Work out the finished part from the listing and answer in its coordinate system (mm). Face numbers are marked on the shaded views. A direction names the side the tool comes from. Coordinates: 2 decimals unless noted, no trailing zeros. Write each loop counter-clockwise with the first axis right and the second up, starting at its lowest first coordinate (ties: lowest second). Pieces come first, ordered by that corner, then holes. Notation, with made-up numbers: M -4.5,-39.75 L 29.5,-39.75 A31 ccw 29.5,-15.75 Z; hole C 4,21 d10. An arc over 180 degrees is marked long. Use CSV: the item, a comma, the result in double quotes.
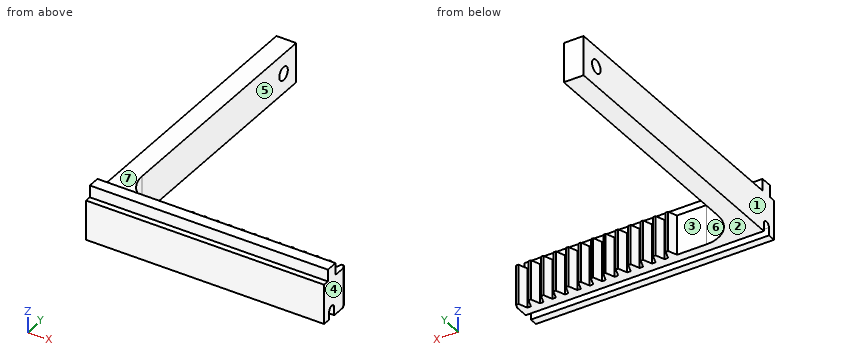
from build123d import *

# Parameters (mm, degrees)
BLANKSKE_W          = 40
BLANKSKE_H          = 8.5
BLANK_DEPTH         = 10
TOOTHCUTSIM_DEPTH   = 43.09809972
TEETHCUTS_COUNT     = 14
TEETHCUTS_PITCH     = 3.14159265
BOSS_EXTRUDE1_DEPTH = 10
SKETCH2_W           = 3
SKETCH2_H           = 3
BOSS_EXTRUDE2_DEPTH = 60
CUT_EXTRUDE2_DEPTH  = 97.566039579
MOVE_FACE2_BY       = 5
FILLET2_R           = 8
SKETCH3_R           = 1.675
CUT_EXTRUDE1_DEPTH  = 94.541434669


with BuildPart() as part:
    # BlankSke → Blank (new body)
    with BuildSketch(Plane.XY):
        with Locations((20, 4.25)):
            Rectangle(BLANKSKE_W, BLANKSKE_H)
    extrude(amount=-BLANK_DEPTH)

    # TooCutSkeSim → ToothCutSim (cut, through all)
    with BuildSketch(Plane.XY):
        Polygon((0.44443537, 6.25), (-0.44443537, 6.25), (-1.272613241, 8.5254), (1.272613241, 8.5254), align=None)
    toothcutsim = extrude(amount=-TOOTHCUTSIM_DEPTH, mode=Mode.SUBTRACT)

    # TeethCuts: ToothCutSim ×14
    with Locations(*[(i * TEETHCUTS_PITCH, 0, 0) for i in range(1, TEETHCUTS_COUNT)]):
        add(toothcutsim, mode=Mode.SUBTRACT)

    # Sketch1 → Boss-Extrude1 (add)
    with BuildSketch(Plane.XY):
        Polygon((0, 0), (-20, 0), (-20, 75), (-10, 75), (-10, 6.25), (0, 6.25), align=None)
    extrude(amount=-BOSS_EXTRUDE1_DEPTH)

    # Sketch2 → Boss-Extrude2 (add)
    with BuildSketch(Plane(origin=(40, 0, 0), x_dir=(0, 0, -1), z_dir=(1, 0, 0))):
        with Locations((-1.5, 3)):
            Rectangle(SKETCH2_W, SKETCH2_H)
    extrude(amount=-BOSS_EXTRUDE2_DEPTH)

    # Sketch5 → Cut-Extrude2 (cut, through all)
    with BuildSketch(Plane(origin=(40, 0, 0), x_dir=(0, 0, -1), z_dir=(1, 0, 0))):
        with BuildLine():
            Line((10, 4), (8, 4))
            ThreePointArc((8, 4), (7, 3), (8, 2))
            Line((8, 2), (10, 2))
            Line((10, 2), (10, 4))
        make_face()
    extrude(amount=-CUT_EXTRUDE2_DEPTH, mode=Mode.SUBTRACT)

    # Move Face2: a face moved inward by 5.0
    extrude(part.faces().sort_by_distance((-10, 40.625, -5))[0], amount=MOVE_FACE2_BY, dir=(-1, 0, 0), mode=Mode.SUBTRACT)

    # Fillet2
    fillet2_edges = [part.edges().sort_by_distance(p)[0] for p in [
        (-15, 6.25, -5),
    ]]
    fillet(fillet2_edges, radius=FILLET2_R)

    # Sketch3 → Cut-Extrude1 (cut, through all)
    with BuildSketch(Plane.ZY.offset(15)):
        with Locations(Location((-5, 70, 0), (0, 0, 90))):
            Circle(SKETCH3_R)
    extrude(amount=CUT_EXTRUDE1_DEPTH, mode=Mode.SUBTRACT)


solid = part.part
Item 1: Consider probe 1 along Z at (x, y) = (-16.65, 70) (3 decimals); probe 2 along Y at (x, z) = (-18.5, -5) (3 decimals); probe 3 along X at (y, z) = (45.5, -4.75). Determine where each line is inside the solid, lowest interval first.
Answer:
probe 1,"z = -10 to -6.675, -3.325 to 0"
probe 2,"y = 0 to 68.325, 71.675 to 75"
probe 3,"x = -20 to -15"
Item 2: Given pin 1 (1.5 mm diameter, centred on x = 8, z = 1, fed in from +Y); pin 2 (2.5 mm diameter, centred on x = 9, z = 2, fed in from -Y); pin 3 (6 mm diameter, centred on x = 14, z = -1, fed in from +Y), each flat-ended and moving along its own axis, determine where each tip first touches the part or whether it passes through.
Answer:
pin 1,"stops at y = 4.5"
pin 2,"stops at y = 1.5"
pin 3,"stops at y = 8.5"
Item 3: The part is cut by section C-C (x = -8.5). Write down the section's boundary in (y, z), then the cut area to 3 significant figures.
Answer:
outline,"M 0,-10 L 2,-10 L 2,-8 A1 cw 4,-8 L 4,-10 L 6.39,-10 L 6.39,0 L 4.5,0 L 4.5,3 L 1.5,3 L 1.5,0 L 0,0 Z"
area,"67.3 mm2"
Item 4: The part is cut by section A-A (y = 70). Write down the section's boundary in (x, z) (3 decimals), then the cut area to 4 significant figures.
Answer:
outline,"M -20,-10 L -15,-10 L -15,-6.675 L -20,-6.675 Z; M -20,-3.325 L -15,-3.325 L -15,0 L -20,0 Z"
area,"33.25 mm2"
Item 5: For a pull along X with two mould halves and no side action, classify the marked faces 1, 2 and 3 as released by +X, released by -X, zero draft, split by the parting line, or undercut.
Answer:
face 1,"released by -X"
face 2,"zero draft"
face 3,"undercut"
Item 6: A tool of negligible diameter and unlimited length cuts with its end or side. For the marked faces 4, 5, 6 and 7, from which of +Z, -Z, +X, -X, +Y, -Y can it reach the whole face along a straight path? Write none if from no direction.
Answer:
face 4,"+Z, -Z, +X, +Y, -Y"
face 5,"+Z, -Z, +X, +Y"
face 6,"+Z, -Z, +Y"
face 7,"+Z, +X, -X, +Y"
Item 7: The part is cut by section B-B (y = 50). Write down the section's boundary in (x, z), then the cut area to 3 significant figures.
Answer:
outline,"M -20,-10 L -15,-10 L -15,0 L -20,0 Z"
area,"50.0 mm2"
Item 8: The part is cut by section D-D (y = 3). Write down the section's boundary in (x, z), then the cut area to 3 significant figures.
Answer:
outline,"M -20,-7 L 40,-7 L 40,3 L -20,3 Z"
area,"600 mm2"
